```python
from build123d import *

# Parameters (mm, degrees)
SKETCH1_R           = 25.25
SKETCH1_R_2         = 1.75
BOSS_EXTRUDE1_DEPTH = 2.4
SKETCH3_R           = 7
BOSS_EXTRUDE3_DEPTH = 11
CUT_EXTRUDE1_DEPTH  = 11
CIRPATTERN1_COUNT   = 12
CHAMFER1_SIZE       = 1
BOSS_EXTRUDE4_START = 8
SKETCH6_R           = 4.749
BOSS_EXTRUDE4_DEPTH = 8
BOSS_EXTRUDE5_START = 8
SKETCH6_3_R         = 3.9
BOSS_EXTRUDE5_DEPTH = 9
CHAMFER2_SIZE       = 1
SKETCH7_W           = 0.3
SKETCH7_H           = 1


with BuildPart() as part:
    # Sketch1 → Boss-Extrude1 (new body)
    with BuildSketch(Plane(origin=(0, 0, 0), x_dir=(1, 0, 0), z_dir=(0, 1, 0))):
        with Locations(Location((0, 0, 0), (0, 0, 270))):
            Circle(SKETCH1_R)
        with Locations(Location((0, 21.75, 0), (0, 0, 270))):
            Circle(SKETCH1_R_2, mode=Mode.SUBTRACT)
        with Locations(Location((-16.661466638, 13.980630511, 0), (0, 0, 270))):
            Circle(SKETCH1_R_2, mode=Mode.SUBTRACT)
        with Locations(Location((16.661466638, 13.980630511, 0), (0, 0, 90))):
            Circle(SKETCH1_R_2, mode=Mode.SUBTRACT)
        with Locations(Location((16.661466638, -13.980630511, 0), (0, 0, 270))):
            Circle(SKETCH1_R_2, mode=Mode.SUBTRACT)
        with Locations(Location((0, -21.75, 0), (0, 0, 90))):
            Circle(SKETCH1_R_2, mode=Mode.SUBTRACT)
        with Locations(Location((-16.661466638, -13.980630511, 0), (0, 0, 90))):
            Circle(SKETCH1_R_2, mode=Mode.SUBTRACT)
    extrude(amount=BOSS_EXTRUDE1_DEPTH)

    # Sketch3 → Boss-Extrude3 (add)
    with BuildSketch(Plane(origin=(0, 2.4, 0), x_dir=(1, 0, 0), z_dir=(0, 1, 0))):
        with Locations(Location((0, 0, 0), (0, 0, 270))):
            Circle(SKETCH3_R)
    extrude(amount=BOSS_EXTRUDE3_DEPTH)

    # Sketch4 → Cut-Extrude1 (cut)
    with BuildSketch(Plane(origin=(0, 13.4, 0), x_dir=(1, 0, 0), z_dir=(0, 1, 0))):
        with BuildLine():
            ThreePointArc((0.562207301, 4.715604304), (0, 4.749), (-0.562207301, 4.715604304))
            ThreePointArc((-0.562207301, 4.715604304), (-0.837528627, 5.917009812), (-1.672850686, 6.823328788))
            ThreePointArc((-1.672850686, 6.823328788), (0, 7.0254), (1.672850686, 6.823328788))
            ThreePointArc((1.672850686, 6.823328788), (0.837528627, 5.917009812), (0.562207301, 4.715604304))
        make_face()
    cut_extrude1 = extrude(amount=-CUT_EXTRUDE1_DEPTH, mode=Mode.SUBTRACT)

    # CirPattern1: Cut-Extrude1 ×12 about axis
    cirpattern1_axis = Axis((0, 0, 0), (0, 1, 0))
    for i in range(1, CIRPATTERN1_COUNT):
        add(cut_extrude1.rotate(cirpattern1_axis, i * 360 / CIRPATTERN1_COUNT), mode=Mode.SUBTRACT)

    # Chamfer1
    chamfer1_edges = [part.edges().sort_by_distance(p)[0] for p in [
        (0, 2.4, -25.25),
    ]]
    chamfer(chamfer1_edges, length=CHAMFER1_SIZE)

    # Sketch6 → Boss-Extrude4 (add)
    with BuildSketch(Plane(origin=(0, 13.4, 0), x_dir=(1, 0, 0), z_dir=(0, 1, 0)).offset(BOSS_EXTRUDE4_START)):
        with Locations(Location((0, 0, 0), (0, 0, 270))):
            Circle(SKETCH6_R)
    extrude(amount=-BOSS_EXTRUDE4_DEPTH)

    # Sketch6<3> → Boss-Extrude5 (add)
    with BuildSketch(Plane(origin=(0, 13.4, 0), x_dir=(1, 0, 0), z_dir=(0, 1, 0)).offset(BOSS_EXTRUDE5_START)):
        with Locations(Location((0, 0, 0), (0, 0, 270))):
            Circle(SKETCH6_3_R)
    extrude(amount=BOSS_EXTRUDE5_DEPTH)

    # Chamfer2
    chamfer2_edges = [part.edges().sort_by_distance(p)[0] for p in [
        (0, 30.4, -3.9),
    ]]
    chamfer(chamfer2_edges, length=CHAMFER2_SIZE)

    # Cut-Sweep1: sweep along a curve in space
    with BuildLine() as cut_sweep1_path:
        ThreePointArc((0, 29.4, 3.9), (2.757716447, 29.4, 2.757716447), (3.9, 29.4, 0))
        ThreePointArc((3.9, 29.4, 0), (2.757716447, 29.4, -2.757716447), (0, 29.4, -3.9))
        ThreePointArc((0, 29.4, -3.9), (-2.757716447, 29.4, -2.757716447), (-3.9, 29.4, 0))
        ThreePointArc((-3.9, 29.4, 0), (-2.757716447, 29.4, 2.757716447), (0, 29.4, 3.9))
    # Sketch7 → Cut-Sweep1 (sweep, cut)
    with BuildSketch(Plane.XY):
        with Locations((-3.75, 26.9)):
            Rectangle(SKETCH7_W, SKETCH7_H)
    sweep(path=cut_sweep1_path.line, mode=Mode.SUBTRACT)


solid = part.part
```
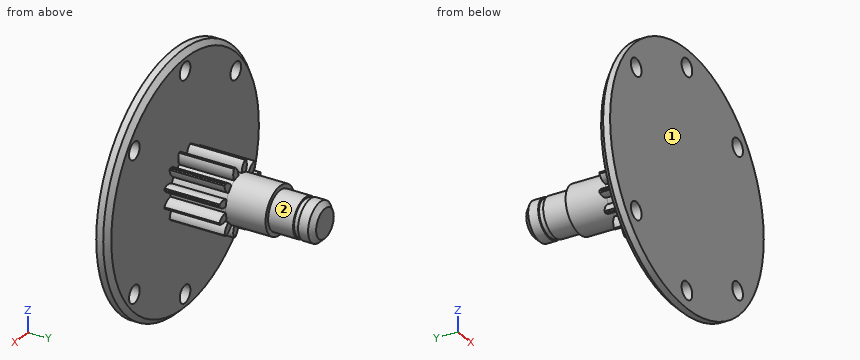
Source: CAD feature listing. Evaluate the final solid. Frame: model axes, mm. Face numbers are marked on the shaded views. A direction names the side the tool comes from. Round coordinates to 2 decimals unless told otherwise and drop trailing zeros. Loops run counter-clockwise (first coordinate to the right, second up) from the corner with the lowest first, then second, coordinate; pieces in that order, holes last. Notation, with made-up numbers: M 18.25,82 L 26.25,82 A29 cw 26.25,108 Z; hole C 42.5,42.5 d8. An arc over 180 degrees is marked long. Put each result on its own line as item: value.
(1) First-contact query: pin 1 (1.8 mm diameter, centred on x = -3.5, z = -4.5, fed in from +Y); pin 2 (12 mm diameter, centred on x = 8.5, y = 21, fed in from +Z); pin 3 (5 mm diameter, centred on x = -6.5, z = -10.5, fed in from +Y); pin 4 (4 mm diameter, centred on x = 0, z = 21.75, fed in from -Y). Flat tips, straight axial feed; report the tip coordinate or a pass-through.
Solutions:
pin 1: y = 13.4
pin 2: z = 4.04
pin 3: y = 2.4
pin 4: y = 0
(2) Section A-A, the plane y = 28.5. Return loops of the section in (x, z), and give its area (3 significant figures).
Solutions:
outline: C 0,0 d7.8
area: 47.8 mm²
(3) Ray query, line 1 (X direction, y = 9.5, z = -2); line 2 (Y direction, x = -5, z = 0); line 3 (X direction, y = 14.5, z = 0). Return the intervals inside material, ascending. Write a range as [from, to].
Solutions:
line 1: [-6.67, -4.6], [-4.31, 4.31], [4.6, 6.67]
line 2: [0, 2.4]
line 3: [-4.75, 4.75]
(4) Section B-B, the plane z = -13.5. State how many separate pieces and enclosed holes the cut face has, and give its area (3 significant figures).
Solutions:
separate pieces: 3
enclosed holes: 0
area: 85.1 mm²
(5) Access query for the marked faces 1 and 2. Directions: +Z, -Z, +X, -X, +Y, -Y. A direction counts if a zero-diameter tool reaches every point of the face in a straight line with its end or side. Return the directions, or none.
Solutions:
face 1: +Z, -Z, +X, -X, -Y
face 2: +Y
